Design review of the part built by this model. Coordinates are the model's own, in mm. A direction names the side the tool comes from. Coordinates: 2 decimals unless noted, no trailing zeros. Loops run counter-clockwise (first coordinate to the right, second up) from the corner with the lowest first, then second, coordinate; pieces in that order, holes last. Notation, with made-up numbers: (32, -3) -> (48, -3) arc R27 ccw to (48, 26) -> close; hole circle Ø7 at (-40, -39.5). An arc over 180 degrees is marked (long way). Answer as a JSON object with one key per item and string values.
```python
from build123d import *

# Parameters (mm, degrees)
SKETCH1_W           = 2.9
SKETCH1_H           = 20
BOSS_EXTRUDE1_DEPTH = 3
FILLET1_R           = 5
FILLET2_R           = 30
CUT_EXTRUDE1_REACH  = 5
SKETCH3_R           = 7.5
SKETCH3_R_2         = 2.3
SKETCH5_W           = 20
SKETCH5_H           = 2.9
CUT_EXTRUDE2_DEPTH  = 3
SKETCH6_R           = 2.3
CUT_EXTRUDE3_DEPTH  = 3


with BuildPart() as part:
    # Sketch1 → Boss-Extrude1 (new body)
    with BuildSketch(Plane.XY):
        Polygon((0, 0), (-23, 0), (-23, 68), (-75, 143), (-47.5, 143), (-47.5, 146), (-27.5, 146), (-27.5, 143), (0, 143), align=None)
        with Locations((-16.5, 15)):
            Rectangle(SKETCH1_W, SKETCH1_H, mode=Mode.SUBTRACT)
        with Locations((-6.5, 15)):
            Rectangle(SKETCH1_W, SKETCH1_H, mode=Mode.SUBTRACT)
    extrude(amount=BOSS_EXTRUDE1_DEPTH)

    # Fillet1
    fillet1_edges = [part.edges().sort_by_distance(p)[0] for p in [
        (0, 0, 1.5),
        (-23, 0, 1.5),
    ]]
    fillet(fillet1_edges, radius=FILLET1_R)

    # Fillet2
    fillet2_edges = [part.edges().sort_by_distance(p)[0] for p in [
        (-23, 68, 1.5),
    ]]
    fillet(fillet2_edges, radius=FILLET2_R)

    # Sketch3 → Cut-Extrude1 (cut, up to next)
    with BuildSketch(Plane(origin=(0, 0, 0), x_dir=(-1, 0, 0), z_dir=(0, 0, -1)), mode=Mode.PRIVATE) as cut_extrude1_sk1:
        with Locations((12, 73)):
            Circle(SKETCH3_R)
    cut_extrude1_tool1 = extrude(cut_extrude1_sk1.sketch, amount=-CUT_EXTRUDE1_REACH, mode=Mode.PRIVATE) & part.part
    add(cut_extrude1_tool1.solids().sort_by_distance((-12, 73, 0))[0], mode=Mode.SUBTRACT)
    # Sketch3 → Cut-Extrude1 (cut, up to next)
    with BuildSketch(Plane(origin=(0, 0, 0), x_dir=(-1, 0, 0), z_dir=(0, 0, -1)), mode=Mode.PRIVATE) as cut_extrude1_sk2:
        with Locations((17.05, 59.5)):
            Circle(SKETCH3_R_2)
    cut_extrude1_tool2 = extrude(cut_extrude1_sk2.sketch, amount=-CUT_EXTRUDE1_REACH, mode=Mode.PRIVATE) & part.part
    add(cut_extrude1_tool2.solids().sort_by_distance((-17.05, 59.5, 0))[0], mode=Mode.SUBTRACT)
    # Sketch3 → Cut-Extrude1 (cut, up to next)
    with BuildSketch(Plane(origin=(0, 0, 0), x_dir=(-1, 0, 0), z_dir=(0, 0, -1)), mode=Mode.PRIVATE) as cut_extrude1_sk3:
        with Locations((6.95, 59.5)):
            Circle(SKETCH3_R_2)
    cut_extrude1_tool3 = extrude(cut_extrude1_sk3.sketch, amount=-CUT_EXTRUDE1_REACH, mode=Mode.PRIVATE) & part.part
    add(cut_extrude1_tool3.solids().sort_by_distance((-6.95, 59.5, 0))[0], mode=Mode.SUBTRACT)
    # Sketch3 → Cut-Extrude1 (cut, up to next)
    with BuildSketch(Plane(origin=(0, 0, 0), x_dir=(-1, 0, 0), z_dir=(0, 0, -1)), mode=Mode.PRIVATE) as cut_extrude1_sk4:
        with Locations((17.05, 109.5)):
            Circle(SKETCH3_R_2)
    cut_extrude1_tool4 = extrude(cut_extrude1_sk4.sketch, amount=-CUT_EXTRUDE1_REACH, mode=Mode.PRIVATE) & part.part
    add(cut_extrude1_tool4.solids().sort_by_distance((-17.05, 109.5, 0))[0], mode=Mode.SUBTRACT)
    # Sketch3 → Cut-Extrude1 (cut, up to next)
    with BuildSketch(Plane(origin=(0, 0, 0), x_dir=(-1, 0, 0), z_dir=(0, 0, -1)), mode=Mode.PRIVATE) as cut_extrude1_sk5:
        with Locations((6.95, 109.5)):
            Circle(SKETCH3_R_2)
    cut_extrude1_tool5 = extrude(cut_extrude1_sk5.sketch, amount=-CUT_EXTRUDE1_REACH, mode=Mode.PRIVATE) & part.part
    add(cut_extrude1_tool5.solids().sort_by_distance((-6.95, 109.5, 0))[0], mode=Mode.SUBTRACT)

    # Sketch5 → Cut-Extrude2 (cut)
    with BuildSketch(Plane(origin=(0, 0, 0), x_dir=(-1, 0, 0), z_dir=(0, 0, -1))):
        with Locations((15, 98)):
            Rectangle(SKETCH5_W, SKETCH5_H)
    extrude(amount=-CUT_EXTRUDE2_DEPTH, mode=Mode.SUBTRACT)

    # Sketch6 → Cut-Extrude3 (cut)
    with BuildSketch(Plane.XY.offset(3)):
        with Locations((-17.05, 39.5)):
            Circle(SKETCH6_R)
        with Locations((-6.95, 39.5)):
            Circle(SKETCH6_R)
    extrude(amount=-CUT_EXTRUDE3_DEPTH, mode=Mode.SUBTRACT)


solid = part.part
```
1) Clearance check with flat-ended pins moving along their axes: pin 1 Ø0.9 at (y, z) = (14, 1.5) entering from -X; pin 2 Ø0.9 at (x, z) = (-6.5, 1.5) entering from +Y; pin 3 Ø1 at (x, z) = (-42.5, 1) entering from -Y; pin 4 Ø6 at (x, y) = (-17.05, 59.5) entering from -Z. State where each tip first meets the part, or that it passes through.
Completed:
{"pin 1": "x = -23", "pin 2": "y = 143", "pin 3": "y = 95.4", "pin 4": "z = 0"}
2) Add section B-B, the plane x = -12. Give the boundary of the cut face in (y, z).
Completed:
{"outline": "(0, 0) -> (65.5, 0) -> (65.5, 3) -> (0, 3) -> close; (80.5, 0) -> (96.55, 0) -> (96.55, 3) -> (80.5, 3) -> close; (99.45, 0) -> (143, 0) -> (143, 3) -> (99.45, 3) -> close"}
3) For faces 4 (the flat face through (-17, 5, 1)), 5 (the flat face through (-47.5, 144, 1)), 6 (the flat face through (-14, 143, 1)), 7 (the flat face through (-11, 0, 1)), list the 3-axis set-ups (+Z, -Z, +X, -X, +Y, -Y) from which the entire face can be reached by the end or side of a thin tool; tool diameter is ignored.
Completed:
{"face 4": "+Z, -Z", "face 5": "+Z, -Z, -X, +Y", "face 6": "+Z, -Z, +X, +Y", "face 7": "+Z, -Z, +X, -X, -Y"}
4) Add section D-D, the plane y = 125. Give the boundary of the cut face in (x, z), and give its area (3 significant figures).
Completed:
{"outline": "(-62.52, 0) -> (0, 0) -> (0, 3) -> (-62.52, 3) -> close", "area": "188 mm²"}
5) Add section C-C, the plane y = 39.5. Give the boundary of the cut face in (x, z).
Completed:
{"outline": "(-23, 0) -> (-19.35, 0) -> (-19.35, 3) -> (-23, 3) -> close; (-14.75, 0) -> (-9.25, 0) -> (-9.25, 3) -> (-14.75, 3) -> close; (-4.65, 0) -> (0, 0) -> (0, 3) -> (-4.65, 3) -> close"}
6) Add section A-A, the plane z = 2. Count the separate pieces of the cut face and the enclosed holes in it, and give its area (3 significant figures).
Completed:
{"separate pieces": "1", "enclosed holes": "10", "area": "4,850 mm²"}
7) Wall thickness on probe 1 along Y at (x, z) = (-12, 1); probe 2 along X at (y, z) = (8, 1.4); probe 3 along X at (y, z) = (53, 2.45): over which ranges is each line inside the solid? List them lowest first.
Completed:
{"probe 1": "0 to 65.5, 80.5 to 96.55, 99.45 to 143", "probe 2": "-23 to -17.95, -15.05 to -7.95, -5.05 to 0", "probe 3": "-23 to 0"}
8) The part is to be moulded in two halves that separate along Y. For faces 1 (the flat face through (-38, 146, 1)), 2 (the flat face through (-23, 31, 1)), 3 (the cylindrical face through (-16.75, 111.78, 1.48)), say which applies: pulls with the +Y half, pulls with the -Y half, needs draft (parallel to the pull), parting line crosses it, or undercut.
Completed:
{"face 1": "pulls with the +Y half", "face 2": "needs draft", "face 3": "undercut"}
